Verification items for the finished model (mm, model axes). Give positions to 0.01 mm unless a question says otherwise; leave off trailing zeros. Order: outer loops, then holes, each group sorted by start corner. A loop starts at its lowest first (then second) coordinate and runs counter-clockwise, first axis right, second up.
(1) Sectioned sample at D-D on x = -44.45. Record the cut outline in (y, z), plus the area to 3 significant figures.
(2) Sectioned sample at B-B on y = 5. Count the separate pieces of the cut face and the enclosed holes in it, plus the area to 3 significant figures.
(3) Sectioned sample at C-C on z = 24.5. Record the cut outline in (x, y).
(4) Sectioned sample at A-A on x = 44. Record the cut outline in (y, z).
(5) Scan lines: L1, parallel to Z at x = -44.45, y = 3.75; L2, parallel to X at y = 2.75, z = 45; L3, parallel to Z at x = 52, y = 3.75. Record each from-to range of solid material in increasing order.
(6) Gauge pin test, flat ends, axial feed: pin 1 (3 mm diameter, centred on y = 2.5, z = 39.5, fed in from -X); pin 2 (4.5 mm diameter, centred on x = 44.45, z = -8.25, fed in from -Y); pin 3 (10 mm diameter, centred on x = 32, z = 37.5, fed in from -Y); pin 4 (1.5 mm diameter, centred on x = 43.5, y = 1, fed in from -Z). Record the tip position at first contact, or that the pin passes through.
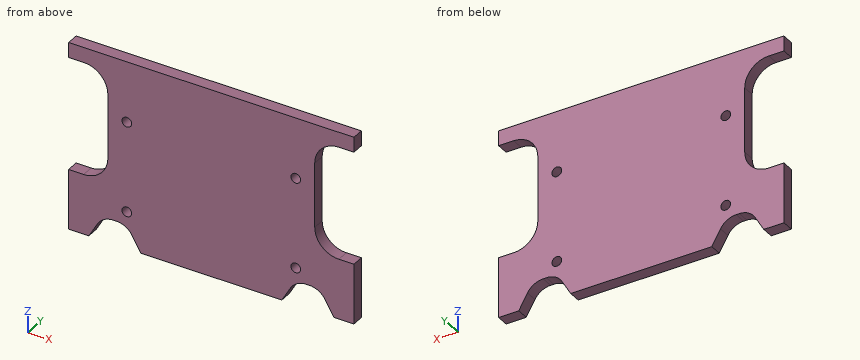
```python
from build123d import *

# Parameters (mm, degrees)
BOSS_EXTRUDE1_DEPTH    = 6.35
F_10_CLEARANCE_HOLE1_D = 5.1054


with BuildPart() as part:
    # Sketch1 → Boss-Extrude1 (new body)
    with BuildSketch(Plane(origin=(0, 0, 0), x_dir=(1, 0, 0), z_dir=(0, 1, 0))):
        with BuildLine():
            Line((-54.448, -16.667265757), (-54.448, -50.812890909))
            ThreePointArc((-54.448, -50.812890909), (-58.167743879, -59.79314703), (-67.148, -63.512890909))
            Line((-67.148, -63.512890909), (-75.0855, -63.512890909))
            Line((-75.0855, -63.512890909), (-75.0855, -71.450390909))
            Line((-75.0855, -71.450390909), (75.0855, -71.450390909))
            Line((75.0855, -71.450390909), (75.0855, -63.512890909))
            Line((75.0855, -63.512890909), (67.148, -63.512890909))
            ThreePointArc((67.148, -63.512890909), (58.167743879, -59.79314703), (54.448, -50.812890909))
            Line((54.448, -50.812890909), (54.448, -16.667265757))
            ThreePointArc((54.448, -16.667265757), (58.167743879, -7.687009636), (67.148, -3.967265757))
            Line((67.148, -3.967265757), (75.0855, -3.967265757))
            Line((75.0855, -3.967265757), (75.0855, 27.782734243))
            Line((75.0855, 27.782734243), (64.482348419, 27.782734243))
            Line((64.482348419, 27.782734243), (59.899630657, 19.845234243))
            ThreePointArc((59.899630657, 19.845234243), (56.413238686, 16.358842272), (51.650738686, 15.082734243))
            Line((51.650738686, 15.082734243), (49.949261314, 15.082734243))
            ThreePointArc((49.949261314, 15.082734243), (45.186761314, 16.358842272), (41.700369343, 19.845234243))
            Line((41.700369343, 19.845234243), (37.117651581, 27.782734243))
            Line((37.117651581, 27.782734243), (-37.117651581, 27.782734243))
            Line((-37.117651581, 27.782734243), (-41.700369343, 19.845234243))
            ThreePointArc((-41.700369343, 19.845234243), (-45.186761314, 16.358842272), (-49.949261314, 15.082734243))
            Line((-49.949261314, 15.082734243), (-51.650738686, 15.082734243))
            ThreePointArc((-51.650738686, 15.082734243), (-56.413238686, 16.358842272), (-59.899630657, 19.845234243))
            Line((-59.899630657, 19.845234243), (-64.482348419, 27.782734243))
            Line((-64.482348419, 27.782734243), (-75.0855, 27.782734243))
            Line((-75.0855, 27.782734243), (-75.0855, -3.967265757))
            Line((-75.0855, -3.967265757), (-67.148, -3.967265757))
            ThreePointArc((-67.148, -3.967265757), (-58.167743879, -7.687009636), (-54.448, -16.667265757))
        make_face()
    extrude(amount=BOSS_EXTRUDE1_DEPTH)

    # #10 Clearance Hole1 (through all)
    with Locations(Plane(origin=(0, 6.35, 0), x_dir=(1, 0, 0), z_dir=(0, 1, 0))):
        with Locations((-44.449999955, 8.251852655), (-44.449999955, -39.373147345), (44.450000045, 8.251852655), (44.450000045, -39.373147345)):
            Hole(F_10_CLEARANCE_HOLE1_D / 2)


solid = part.part
```
Ans:
1. outline: (0, -16.83) - (6.35, -16.83) - (6.35, -10.8) - (0, -10.8) - close; (0, -5.7) - (6.35, -5.7) - (6.35, 36.82) - (0, 36.82) - close; (0, 41.93) - (6.35, 41.93) - (6.35, 71.45) - (0, 71.45) - close
1. area: 496 mm2
2. separate pieces: 1
2. enclosed holes: 4
2. area: 12,000 mm2
3. outline: (-54.45, 0) - (54.45, 0) - (54.45, 6.35) - (-54.45, 6.35) - close
4. outline: (0, -17.17) - (6.35, -17.17) - (6.35, -10.76) - (0, -10.76) - close; (0, -5.74) - (6.35, -5.74) - (6.35, 36.86) - (0, 36.86) - close; (0, 41.89) - (6.35, 41.89) - (6.35, 71.45) - (0, 71.45) - close
5. L1: z = -16.83 to -10.8, -5.7 to 36.82, 41.93 to 71.45
5. L2: x = -54.45 to 54.45
5. L3: z = -15.09 to 71.45
6. pin 1: stops at x = -54.45
6. pin 2: passes through
6. pin 3: stops at y = 0
6. pin 4: stops at z = -18.37
